```python
from build123d import *
from build123d.topology import SkipClean

# Parameters (mm, degrees)
SKETCH1_R           = 15.875
BOSS_EXTRUDE1_DEPTH = 4.7625
BOSS_EXTRUDE2_DEPTH = 25.4
FILLET1_R           = 0.508


with BuildPart() as part:
    # Sketch1 → Boss-Extrude1 (new body)
    with BuildSketch(Plane.XY):
        with Locations(Location((0, 0, 0), (0, 0, 180))):
            Circle(SKETCH1_R)
        Polygon((5.719231767, 0), (2.859615883, 4.953), (-2.859615883, 4.953), (-5.719231767, 0), (-2.859615883, -4.953), (2.859615883, -4.953), align=None, mode=Mode.SUBTRACT)
    extrude(amount=BOSS_EXTRUDE1_DEPTH)

    # Sketch2 → Boss-Extrude2 (add)
    with SkipClean():  # the faces are left unmerged after this step: merging them gives an invalid solid
        with BuildSketch(Plane.XY.offset(4.7625)):
            with BuildLine():
                Line((-15.875, 0), (-14.605, 0))
                ThreePointArc((-14.605, 0), (-5.58909153, 13.493260572), (10.327294539, 10.327294539))
                Line((10.327294539, 10.327294539), (11.225320151, 11.225320151))
                ThreePointArc((11.225320151, 11.225320151), (-6.075099489, 14.666587579), (-15.875, 0))
            make_face()
        extrude(amount=BOSS_EXTRUDE2_DEPTH)

    # Fillet1
    fillet1_edges = [part.edges().sort_by_distance(p)[0] for p in [
        (-14.605, 0, 17.4625),
        (10.327294539, 10.327294539, 17.4625),
    ]]
    fillet(fillet1_edges, radius=FILLET1_R)


solid = part.part
```
Model file for the job. Use its own axes, mm. A direction names the side the tool comes from. Round coordinates to 2 decimals unless told otherwise and drop trailing zeros. Write each loop counter-clockwise with the first axis right and the second up, starting at its lowest first coordinate (ties: lowest second). Pieces come first, ordered by that corner, then holes. Notation, with made-up numbers: (68, 13.5) - (83, 13.5) arc R14 ccw to (83, 18.5) - close; hole circle Ø7 at (-16.5, 39). An arc over 180 degrees is marked (long way). Use CSV: the item, a comma, the result in double quotes. Start each with the question number.
Item 1: Two-plate mould, pull along Y, no slides. Class faces 1 (the face through (0, -4.953, 2)), 2 (the face through (-5.805, 13.402, 17.285)), 3 (the face through (4, -4, 0)): released by +Y, released by -Y, zero draft, split by the parting line, or undercut.
Item 2: Band-saw the part on C-C (x = -9.5). Write the cut outline in (y, z), and give its area (3 significant figures).
Item 3: Pin check, flat tips, straight feed: P1, Ø1.5, axis at y = 8.5, z = 18, coming from the -X side; P2, Ø9, axis at x = 6, y = -1, coming from the +Z side; P3, Ø2, axis at y = 1.5, z = 11, coming from the +X side; P4, Ø6, axis at y = -4.5, z = 10.5, coming from the -X side. Stop position of each tip, or through.
Item 4: Band-saw the part on B-B (y = 3). Write the cut outline in (x, z), and give its area (3 significant figures).
Item 5: Band-saw the part on A-A (x = 0). Write the cut outline in (y, z) (1 decimal), and give its area (3 significant figures).
Item 6: Drill centre lines: L1, parallel to Z at x = -3, y = 6; L2, parallel to X at y = 3, z = 22.5; L3, parallel to Y at x = 6, z = 26. Where is each one in solid material? Low to high. Write a range as [from, to].
Item 7: Band-saw the part on D-D (y = 6.5). Write the cut outline in (x, z), and give its area (3 significant figures).
Item 8: Tool access for faces 4 (the face through (-6.4, 13.3, 30.162)), 5 (the face through (0, 4.953, 2)): list every direction of +Z, -Z, +X, -X, +Y, -Y with a clear straight run to the whole face (end or side of a thin tool).
Checked values:
1,face 1,"undercut"
1,face 2,"released by -Y"
1,face 3,"zero draft"
2,outline,"(-12.72, 0) - (12.72, 0) - (12.72, 30.16) - (11.09, 30.16) - (11.09, 4.76) - (-12.72, 4.76) - close"
2,area,"162 mm²"
3,P1,"stops at x = -13.85"
3,P2,"stops at z = 4.76"
3,P3,"stops at x = -14.39"
3,P4,"passes through"
4,outline,"(-15.59, 0) - (-3.99, 0) - (-3.99, 4.76) - (-14.29, 4.76) - (-14.29, 30.16) - (-15.59, 30.16) - close; (3.99, 0) - (15.59, 0) - (15.59, 4.76) - (3.99, 4.76) - close"
4,area,"143 mm²"
5,outline,"(-15.9, 0) - (-5, 0) - (-5, 4.8) - (-15.9, 4.8) - close; (5, 0) - (15.9, 0) - (15.9, 30.2) - (14.6, 30.2) - (14.6, 4.8) - (5, 4.8) - close"
5,area,"136 mm²"
6,L1,"z = [0, 4.76]"
6,L2,"x = [-15.59, -14.29]"
6,L3,"y = [13.32, 14.7]"
7,outline,"(-14.48, 0) - (14.48, 0) - (14.48, 4.76) - (-13.08, 4.76) - (-13.08, 30.16) - (-14.48, 30.16) - close"
7,area,"174 mm²"
8,face 4,"+Z, +X, -X, +Y, -Y"
8,face 5,"+Z, -Z"
